from build123d import *
from build123d import SkipClean  # not in build123d's __all__

# Parameters (mm, degrees)
F1_DEPTH  = 25
F2_R      = 0.5
F3_DEPTH  = 1
F4_R      = 2.5
F4_R_2    = 0.5
F5_DEPTH  = 2
F7_DEPTH  = 1
F9_DEPTH  = 1
F11_DEPTH = 1
F12_DEPTH = 1
F14_DEPTH = 1


# Not quite as in the source:
# - a feature names something its author has since deleted; it is built from what else it names


with BuildPart() as f1:
    # F0 (on Top) → F1 (new body)
    with BuildSketch(Plane.XY):
        with BuildLine():
            Line((-8.65676943, -0.5), (-1.4142135624, -0.5))
            ThreePointArc((-1.4142135624, -0.5), (-1.0606601718, -1.0606601718), (-0.5, -1.4142135624))
            Line((-0.5, -1.4142135624), (-0.5, -8.65676943))
            Line((-0.5, -8.65676943), (0.5, -8.65676943))
            Line((0.5, -8.65676943), (0.5, -1.4142135624))
            ThreePointArc((0.5, -1.4142135624), (1.0606601718, -1.0606601718), (1.4142135624, -0.5))
            Line((1.4142135624, -0.5), (8.65676943, -0.5))
            Line((8.65676943, -0.5), (8.65676943, 0.5))
            Line((8.65676943, 0.5), (1.4142135624, 0.5))
            ThreePointArc((1.4142135624, 0.5), (1.0606601718, 1.0606601718), (0.5, 1.4142135624))
            Line((0.5, 1.4142135624), (0.5, 8.65676943))
            Line((0.5, 8.65676943), (-0.5, 8.65676943))
            Line((-0.5, 8.65676943), (-0.5, 1.4142135624))
            ThreePointArc((-0.5, 1.4142135624), (-1.0606601718, 1.0606601718), (-1.4142135624, 0.5))
            Line((-1.4142135624, 0.5), (-8.65676943, 0.5))
            Line((-8.65676943, 0.5), (-8.65676943, -0.5))
        make_face()
        with BuildLine():
            ThreePointArc((0, 0.5), (0.3535533906, 0.3535533906), (0.5, 0))
            ThreePointArc((0.5, 0), (-0.3535533906, -0.3535533906), (0, 0.5))
        make_face(mode=Mode.SUBTRACT)
    extrude(amount=F1_DEPTH)

    # F2 (on face) → F3 (join)
    with BuildSketch(Plane.XY.offset(25)):
        with BuildLine():
            ThreePointArc((1.4142135624, -0.5), (1.4783978395, -0.2536529681), (1.5, 0))
            ThreePointArc((1.5, 0), (1.4783978395, 0.2536529681), (1.4142135624, 0.5))
            ThreePointArc((1.4142135624, 0.5), (1.0606601718, 1.0606601718), (0.5, 1.4142135624))
            ThreePointArc((0.5, 1.4142135624), (0, 1.5), (-0.5, 1.4142135624))
            ThreePointArc((-0.5, 1.4142135624), (-1.0606601718, 1.0606601718), (-1.4142135624, 0.5))
            ThreePointArc((-1.4142135624, 0.5), (-1.5, 0), (-1.4142135624, -0.5))
            ThreePointArc((-1.4142135624, -0.5), (-1.0606601718, -1.0606601718), (-0.5, -1.4142135624))
            ThreePointArc((-0.5, -1.4142135624), (0, -1.5), (0.5, -1.4142135624))
            ThreePointArc((0.5, -1.4142135624), (1.0606601718, -1.0606601718), (1.4142135624, -0.5))
        make_face()
        Circle(F2_R, mode=Mode.SUBTRACT)
    with SkipClean():  # cleaning this boolean's faces spoils the solid; the shape is the same uncleaned
        extrude(amount=F3_DEPTH)

    # F4 (on face) → F5 (join)
    with BuildSketch(Plane(origin=(0, 0, 0), x_dir=(1, 0, 0), z_dir=(0, 0, -1))):
        Circle(F4_R)
        Circle(F4_R_2, mode=Mode.SUBTRACT)
    extrude(amount=-F5_DEPTH)

    # F6 (on face) → F7 (join)
    with BuildSketch(Plane.YZ.offset(0.5)):
        with BuildLine():
            Line((-8.65676943, 0), (-8.65676943, 25))
            ThreePointArc((-8.65676943, 25), (-21.15676943, 12.5), (-8.65676943, 0))
        make_face()
    extrude(amount=-F7_DEPTH)

    # F8 (on face) → F9 (join)
    with BuildSketch(Plane(origin=(0, 0.5, 0), x_dir=(-1, 0, 0), z_dir=(0, 1, 0))):
        with BuildLine():
            Line((8.65676943, 25), (8.65676943, 0))
            ThreePointArc((8.65676943, 0), (21.15676943, 12.5), (8.65676943, 25))
        make_face()
    extrude(amount=-F9_DEPTH)

    # F10 (on face) → F11 (join)
    with BuildSketch(Plane(origin=(-0.5, 0, 0), x_dir=(0, -1, 0), z_dir=(-1, 0, 0))):
        with BuildLine():
            Line((-8.65676943, 0), (-8.65676943, 25))
            ThreePointArc((-8.65676943, 25), (-21.15676943, 12.5), (-8.65676943, 0))
        make_face()
    extrude(amount=-F11_DEPTH)


with BuildPart() as f12:
    # F12 (new): a face of the model
    f12_faces = [f1.part.faces().sort_by_distance(p)[0] for p in [
        (5.0713936624, 0.5, 12.63302926),
    ]]
    extrude(f12_faces, amount=-F12_DEPTH)


with BuildPart() as f1_1:
    add(f1.part, clean=False)

    add(f12.part)  # F14 merges F12
    # F13 (on face) → F14 (join)
    with BuildSketch(Plane(origin=(0, 0.5, 0), x_dir=(-1, 0, 0), z_dir=(0, 1, 0))):
        with BuildLine():
            Line((-8.65676943, 0), (-8.65676943, 25))
            ThreePointArc((-8.65676943, 25), (-21.15676943, 12.5), (-8.65676943, 0))
        make_face()
    extrude(amount=-F14_DEPTH)


solid = f1_1.part
Can you work these out from the model? Positions are in its coordinate system, mm. A direction names the side the tool comes from. Give positions to 0.01 mm unless a question says otherwise; leave off trailing zeros. Loops run counter-clockwise (first coordinate to the right, second up) from the corner with the lowest first, then second, coordinate; pieces in that order, holes last. Notation, with made-up numbers: (18, 85) -> (34, 85) arc R32 ccw to (34, 124) -> close; hole circle Ø10 at (-21, -31). An arc over 180 degrees is marked (long way). Write item = value, one per line.
1) Will these pins go through, and if not, where does the flat tip stop? pin 1 (0.9 mm diameter, centred on x = 0, y = 0, fed in from -Z); pin 2 (2 mm diameter, centred on x = 13.5, z = 4, fed in from +Y); pin 3 (10 mm diameter, centred on x = -11, z = 11.5, fed in from -Y); pin 4 (1.5 mm diameter, centred on x = 1, z = 8.5, fed in from +Y).
Check result:
pin_1 = through
pin_2 = 0.5
pin_3 = -0.5
pin_4 = 20.67
2) I need wall thicknesses on L1, parallel to Y at x = 0, z = 25.2; L2, parallel to X at y = 5.5, z = 18.25. Which ranges of each line are inside material? Lowest first, please. Write a range as from..to.
Check result:
L1 = -1.5..-0.5, 0.5..1.5
L2 = -0.5..0.5
3) Suppose I cut it at B-B on x = 8. Write out the boundary of the cut face in (y, z), then the cut area to 3 significant figures.
Check result:
outline = (-0.5, 0) -> (0.5, 0) -> (0.5, 25) -> (-0.5, 25) -> close
area = 25.0 mm2
4) Suppose I cut it at D-D on y = 16.5. Write out the boundary of the cut face in (x, z), then the cut area to 3 significant figures.
Check result:
outline = (-0.5, 2.77) -> (0.5, 2.77) -> (0.5, 22.23) -> (-0.5, 22.23) -> close
area = 19.5 mm2
5) Suppose I cut it at A-A on z = 12.5. Write out the boundary of the cut face in (x, y).
Check result:
outline = (-21.16, -0.5) -> (-1.41, -0.5) arc R1.5 ccw to (-0.5, -1.41) -> (-0.5, -21.16) -> (0.5, -21.16) -> (0.5, -1.41) arc R1.5 ccw to (1.41, -0.5) -> (21.16, -0.5) -> (21.16, 0.5) -> (1.41, 0.5) arc R1.5 ccw to (0.5, 1.41) -> (0.5, 21.16) -> (-0.5, 21.16) -> (-0.5, 1.41) arc R1.5 ccw to (-1.41, 0.5) -> (-21.16, 0.5) -> close; hole circle Ø1 at (0, 0)
6) Suppose I cut it at C-C on z = 21.5. Write out the boundary of the cut face in (x, y).
Check result:
outline = (-17.33, -0.5) -> (-1.41, -0.5) arc R1.5 ccw to (-0.5, -1.41) -> (-0.5, -17.33) -> (0.5, -17.33) -> (0.5, -1.41) arc R1.5 ccw to (1.41, -0.5) -> (17.33, -0.5) -> (17.33, 0.5) -> (1.41, 0.5) arc R1.5 ccw to (0.5, 1.41) -> (0.5, 17.33) -> (-0.5, 17.33) -> (-0.5, 1.41) arc R1.5 ccw to (-1.41, 0.5) -> (-17.33, 0.5) -> close; hole circle Ø1 at (0, 0)
7) For faces 1 (the flat face through (1.5, 1.5, 2)), 2 (the flat face through (1.5, -1.5, 2)), 3 (the flat face through (-1.5, 1.5, 2)), 4 (the cylindrical face through (0.007, -21.154, 12.775)), 5 (the flat face through (-1.5, -1.5, 2)), which set-ups out of +Z, -Z, +X, -X, +Y, -Y let a thin tool reach every point of the face, with its end or its side?
Check result:
face_1 = +Z, +X, +Y
face_2 = +Z, +X, -Y
face_3 = +Z, -X, +Y
face_4 = +X, -X, -Y
face_5 = +Z, -X, -Y
